from build123d import *

# Parameters (mm, degrees)
F0_W     = 95
F0_H     = 95
F1_DEPTH = 900
F2_W     = 95
F2_H     = 95
F2_W_2   = 70
F2_H_2   = 70
F3_DEPTH = 170


with BuildPart() as f1:
    # F0 (on Top) → F1 (new body)
    with BuildSketch(Plane.XY):
        Rectangle(F0_W, F0_H)
    extrude(amount=-F1_DEPTH)

    # F2 (on face) → F3 (cut)
    with BuildSketch(Plane(origin=(0, 0, -900), x_dir=(1, 0, 0), z_dir=(0, 0, -1))):
        Rectangle(F2_W, F2_H)
        Rectangle(F2_W_2, F2_H_2, mode=Mode.SUBTRACT)
    extrude(amount=-F3_DEPTH, mode=Mode.SUBTRACT)


solid = f1.part
Work out the finished part from the listing and answer in its coordinate system (mm). A direction names the side the tool comes from. Round coordinates to 2 decimals unless told otherwise and drop trailing zeros. Order: outer loops, then holes, each group sorted by start corner. A loop starts at its lowest first (then second) coordinate and runs counter-clockwise, first axis right, second up. Notation, with made-up numbers: M 49.25,58 L 64.25,58 A21 cw 64.25,77 Z; hole C -13,28.5 d2. An arc over 180 degrees is marked long. One line per item, written item: value.
Q1. Determine the mould class of faces 1 (the face through (0, 35, -816)), 2 (the face through (-1, -47.5, -360)), 3 (the face through (-1, 1, 0)) for opening direction Y: released by +Y, released by -Y, zero draft, split by the parting line, or undercut.
Derived:
face 1: released by +Y
face 2: released by -Y
face 3: zero draft
Q2. For faces 4 (the face through (0, -35, -816)), 5 (the face through (-35, 0, -816)), 6 (the face through (47.5, -1, -360)), 7 (the face through (35, 0, -816)), 8 (the face through (0, 0, -900)), determine the directions among +Z, -Z, +X, -X, +Y, -Y from which every point of the face is accessible in a straight line to the end or side of a thin tool.
Derived:
face 4: -Z, +X, -X, -Y
face 5: -Z, -X, +Y, -Y
face 6: +Z, -Z, +X, +Y, -Y
face 7: -Z, +X, +Y, -Y
face 8: -Z, +X, -X, +Y, -Y
Q3. Straight lines are drawn through the part: line 1 (Z direction, x = 25, y = 38); line 2 (X direction, y = -32.5, z = -815). For each, find the intervals that lie inside material, in ascending order.
Derived:
line 1: -730 to 0
line 2: -35 to 35
Q4. Flat-ended cylindrical pins translate along their axes: pin 1 (21 mm diameter, centred on x = -6, z = -801.5, fed in from +Y); pin 2 (21 mm diameter, centred on y = -9, z = -832.5, fed in from -X). Find the tip coordinate at first contact, or state that the pin passes through.
Derived:
pin 1: y = 35
pin 2: x = -35
Q5. Find section A-A on x = 9.5. Write down the section's boundary in (y, z), then the cut area to 4 significant figures.
Derived:
outline: M -47.5,-730 L -35,-730 L -35,-900 L 35,-900 L 35,-730 L 47.5,-730 L 47.5,0 L -47.5,0 Z
area: 81,250 mm²
